```python
from build123d import *

# Parameters (mm, degrees)
F0_W     = 127
F0_H     = 127
F1_DEPTH = 127
F2_R     = 38.1
F3_DEPTH = 127.001
F4_R     = 38.1
F5_DEPTH = 127.001
F6_R     = 38.1
F7_DEPTH = 127.001


with BuildPart() as f1:
    # F0 (on Top) → F1 (new body)
    with BuildSketch(Plane.XY):
        with Locations((6.54018, 6.704748)):
            Rectangle(F0_W, F0_H)
    extrude(amount=F1_DEPTH)

    # F2 (on face) → F3 (cut, through all)
    with BuildSketch(Plane.XY.offset(127)):
        with Locations((6.54018, 6.704748)):
            Circle(F2_R)
    extrude(amount=-F3_DEPTH, mode=Mode.SUBTRACT)

    # F4 (on face) → F5 (cut, through all)
    with BuildSketch(Plane.YZ.offset(70.04018)):
        with Locations((6.704748, 62.066816)):
            Circle(F4_R)
    extrude(amount=-F5_DEPTH, mode=Mode.SUBTRACT)

    # F6 (on face) → F7 (cut, through all)
    with BuildSketch(Plane.XZ.offset(56.795252)):
        with Locations((6.54018, 63.5)):
            Circle(F6_R)
    extrude(amount=-F7_DEPTH, mode=Mode.SUBTRACT)


solid = f1.part
```
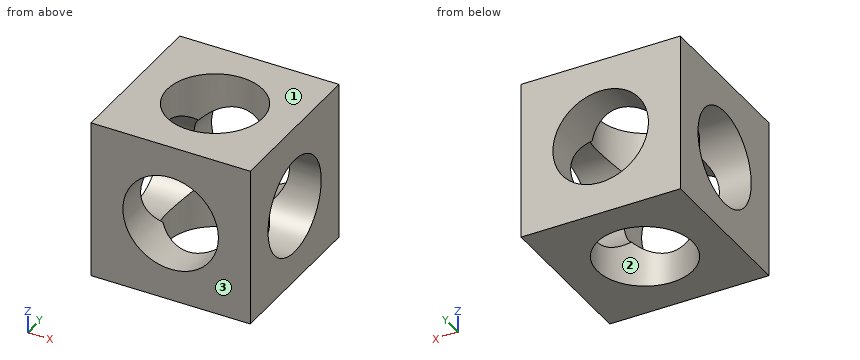
Part model, mm, in its own coordinate system. Face numbers are marked on the shaded views. Round coordinates to 2 decimals unless told otherwise and drop trailing zeros. Loops run counter-clockwise (first coordinate to the right, second up) from the corner with the lowest first, then second, coordinate; pieces in that order, holes last.
Item 1: Cut at A-A, the plane y = 0. Give the cut face in (x, z), then the cut area to 3 significant figures.
Item 2: Cut at B-B, the plane z = 40.5. Give the cut face in (x, y).
Item 3: Mould opens along Y. For the marked faces 1, 2 and 3 say: +Y half, -Y half, draft (parallel to the pull), parting line (faces both ways), or undercut.
Item 4: Drill centre lines: line 1 (X direction, y = 51, z = 63); line 2 (Y direction, x = 28.5, z = 111.5); line 3 (Z direction, x = 32.5, y = -30). Where is each one in solid material? Low to high.
Item 5: Cut at C-C, the plane z = 118. Give the cut face in (x, y).
A:
1. outline: (-56.96, 0) - (-30.97, 0) - (-30.97, 24.56) - (-56.96, 24.56) - close; (-56.96, 99.57) - (-30.97, 99.57) - (-30.97, 127) - (-56.96, 127) - close; (44.05, 0) - (70.04, 0) - (70.04, 24.56) - (44.05, 24.56) - close; (44.05, 99.57) - (70.04, 99.57) - (70.04, 127) - (44.05, 127) - close
1. area: 2,700 mm2
2. outline: (-56.96, -56.8) - (-23.83, -56.8) - (-23.83, -24.7) - (-56.96, -24.7) - close; (-56.96, 38.11) - (-23.83, 38.11) - (-23.83, 70.2) - (-56.96, 70.2) - close; (36.91, -56.8) - (70.04, -56.8) - (70.04, -24.7) - (36.91, -24.7) - close; (36.91, 38.11) - (70.04, 38.11) - (70.04, 70.2) - (36.91, 70.2) - close
3. face 1: draft
3. face 2: undercut
3. face 3: -Y half
4. line 1: x = -56.96 to -31.56, 44.64 to 70.04
4. line 2: y = -56.8 to -24.43, 37.84 to 70.2
4. line 3: z = 0 to 35.61, 91.39 to 127
5. outline: (-56.96, -56.8) - (70.04, -56.8) - (70.04, 70.2) - (-56.96, 70.2) - close; hole circle Ø76.2 at (6.54, 6.7)
